Read the model definition and answer for the solid it produces. Units are mm, in the model's axes. A direction names the side the tool comes from. Round coordinates to 2 decimals unless told otherwise and drop trailing zeros. Order: outer loops, then holes, each group sorted by start corner. A loop starts at its lowest first (then second) coordinate and runs counter-clockwise, first axis right, second up. Notation, with made-up numbers: (11, -2.75) -> (27, -2.75) arc R12 cw to (27, 14.25) -> close; hole circle Ø6 at (54, 51.25). An arc over 180 degrees is marked (long way). Use a Markdown table: item, result. Add a question column.
1. For faces 4 (the face through (19, 0, -2)), 5 (the face through (0.986, 0.74, 1.305)), 6 (the face through (0, -1.3, -1.3)), determine the directions among +Z, -Z, +X, -X, +Y, -Y from which every point of the face is accessible in a straight line to the end or side of a thin tool.
2. Given pin 1 (1 mm diameter, centred on x = 11.5, z = 2, fed in from +Y); pin 2 (2 mm diameter, centred on x = 9, z = 2, fed in from -Y); pin 3 (4 mm diameter, centred on x = 25.5, y = -1, fed in from -Z); pin 4 (3.5 mm diameter, centred on y = 0.5, z = -0.5, fed in from -X), each flat-ended and moving along its own axis, determine where each tip first touches the part or whether it passes through.
3. The mould has two halves that part along Y. Classify faces 1 (the face through (2, 0, 0)), 2 (the face through (33.91, 0, 0)), 3 (the face through (2.229, 3.233, -1.341)): +Y half, -Y half, draft (parallel to the pull), parting line (faces both ways), or undercut.
4. Section A-A, the plane z = 0 is taken. Give the vertices of the cut face in (x, y).
5. Section B-B, the plane x = 17 is taken. Give the vertices of the cut face in (y, z).
6. Consider L1, parallel to X at y = 2.25, z = 1.25; L2, parallel to X at y = 0.5, z = 0.5; L3, parallel to Z at x = 21, y = 0. Determine where each line is inside the solid, lowest interval first. Write a range as [from, to].
```python
from build123d import *

# Parameters (mm, degrees)
CUT_EXTRUDE_1_DEPTH = 2
FILLET_1_R          = 0.5


with BuildPart() as part:
    # 草图1 → 旋转1 (revolve)
    with BuildSketch(Plane.XY):
        Polygon((0, 0), (0, 3.5), (3.91, 3.5), (3.91, 2), (33.91, 2), (33.91, 0), align=None)
    revolve(axis=Axis((0, 0, 0), (1, 0, 0)))

    # 草图2 → 切除-拉伸1 (cut)
    with BuildSketch(Plane.ZY):
        Polygon((-1.732050808, 0), (-0.866025404, -1.5), (0.866025404, -1.5), (1.732050808, 0), (0.866025404, 1.5), (-0.866025404, 1.5), align=None)
    extrude(amount=-CUT_EXTRUDE_1_DEPTH, mode=Mode.SUBTRACT)

    # 圆角1
    fillet_1_edges = [part.edges().sort_by_distance(p)[0] for p in [
        (0, -3.5, 0),
    ]]
    fillet(fillet_1_edges, radius=FILLET_1_R)


solid = part.part
```
Verdict:
| question | item | result |
|---|---|---|
| 1 | face 4 | +X |
| 1 | face 5 | -X |
| 1 | face 6 | +Z, -Z, -X, +Y, -Y |
| 2 | pin 1 | stops at y = 1.32 |
| 2 | pin 2 | stops at y = -1.73 |
| 2 | pin 3 | stops at z = -2 |
| 2 | pin 4 | stops at x = 0 |
| 3 | face 1 | undercut |
| 3 | face 2 | draft |
| 3 | face 3 | parting line |
| 4 | outline | (0, -3) arc R0.5 ccw to (0.5, -3.5) -> (3.91, -3.5) -> (3.91, -2) -> (33.91, -2) -> (33.91, 2) -> (3.91, 2) -> (3.91, 3.5) -> (0.5, 3.5) arc R0.5 ccw to (0, 3) -> (0, 1.5) -> (2, 1.5) -> (2, -1.5) -> (0, -1.5) -> close |
| 5 | outline | circle Ø4 at (0, 0) |
| 6 | L1 | x = [0, 3.91] |
| 6 | L2 | x = [2, 33.91] |
| 6 | L3 | z = [-2, 2] |
